Design review of the part shown in the three views and the two pictorial views. Dimensions are in mm from the part's minimum x, y and z. A direction names the side the tool comes from. Give positions to 0.01 mm unless a question says otherwise; leave off trailing zeros. Order: outer loops, then holes, each group sorted by start corner. A loop starts at its lowest first (then second) coordinate and runs counter-clockwise, first axis right, second up. Notation, with made-up numbers: (56, 52) -> (83, 52) arc R3 ccw to (83, 57) -> close; hole circle Ø10 at (60, -15). An arc over 180 degrees is marked (long way). Use one line per item in the form item = value.
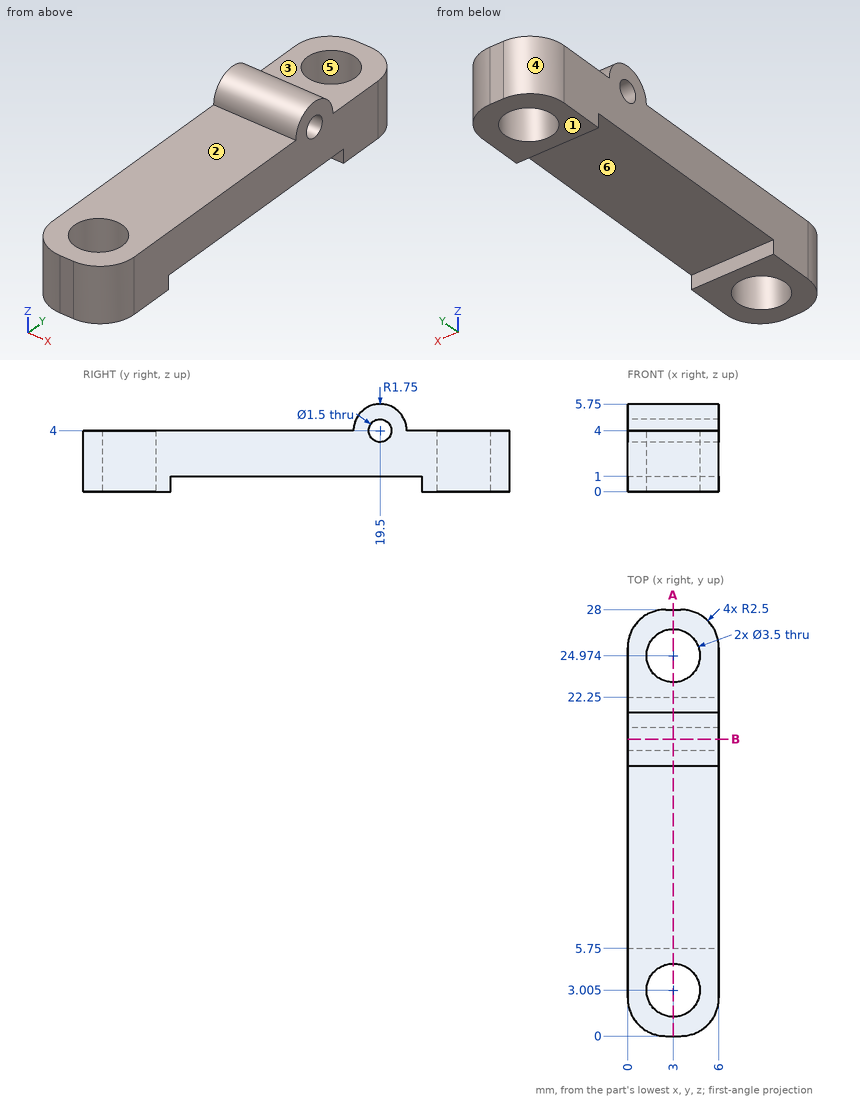
1. For pin 1 Ø1.1 at (x, z) = (1.5, 0.5) entering from +Y; pin 2 Ø1.5 at (x, y) = (1, 8.5) entering from -Z, all flat-tipped, find the tip position at first contact; note any pin that passes through.
Values:
pin_1 = 27.96
pin_2 = 1
2. Tool access review of the marked faces 1, 2 and 3: name each direction out of +Z, -Z, +X, -X, +Y, -Y from which nothing blocks a thin tool from reaching the whole face with its end or side.
Values:
face_1 = -Z, +X, -X, +Y, -Y
face_2 = +Z, +X, -X, -Y
face_3 = +Z, +X, -X, +Y
3. Add section A-A on x = 3. Count the separate pieces of the cut face and the enclosed holes in it.
Values:
separate_pieces = 3
enclosed_holes = 1
4. For L1, parallel to Y at x = 4, z = 3.5; L2, parallel to Y at x = 3, z = 2.5 (1 decimal); L3, parallel to Y at x = 4, z = 0.9, list the stretches that pass through material, from the lowest coordinate up.
Values:
L1 = 0.05 to 1.57, 4.44 to 18.94, 20.06 to 23.54, 26.41 to 27.95
L2 = 0 to 1.3, 4.8 to 23.2, 26.7 to 28
L3 = 0.05 to 1.57, 4.44 to 5.75, 22.25 to 23.54, 26.41 to 27.95
5. Add section B-B on y = 19.5. Give the boundary of the cut face in (x, z), then the cut area to 3 significant figures.
Values:
outline = (0, 1) -> (6, 1) -> (6, 3.25) -> (0, 3.25) -> close; (0, 4.75) -> (6, 4.75) -> (6, 5.75) -> (0, 5.75) -> close
area = 19.5 mm^2
6. The part is to be moulded in two halves that separate along X. For the marked faces 4, 5 and 6, say which applies: +X half, -X half, draft (parallel to the pull), parting line (faces both ways), or undercut.
Values:
face_4 = -X half
face_5 = undercut
face_6 = draft
